```python
from build123d import *

# Parameters (mm, degrees)
F0_R     = 9.5
F1_DEPTH = 10


with BuildPart() as f1:
    # F0 (on Top) → F1 (new body)
    with BuildSketch(Plane.XY):
        with BuildLine():
            Line((0.545393, 36.038877), (-22.02152, 29.448028))
            ThreePointArc((-22.02152, 29.448028), (-26.833244, 26.063712), (-28.572816, 20.444089))
            Line((-28.572816, 20.444089), (-27.988367, 0.026176))
            ThreePointArc((-27.988367, 0.026176), (-27.827538, -1.655225), (-27.444354, -3.300261))
            Line((-27.444354, -3.300261), (-21.763491, -21.955443))
            ThreePointArc((-21.763491, -21.955443), (-21.078383, -23.186097), (-19.947006, -24.025066))
            Line((-19.947006, -24.025066), (-0.808983, -32.702572))
            ThreePointArc((-0.808983, -32.702572), (1.170286, -33.37879), (3.242493, -33.662925))
            Line((3.242493, -33.662925), (22.94121, -34.447196))
            ThreePointArc((22.94121, -34.447196), (23.121499, -34.452579), (23.30186, -34.454373))
            Line((23.30186, -34.454373), (30.367569, -34.454373))
            ThreePointArc((30.367569, -34.454373), (31.781783, -33.868586), (32.367569, -32.454373))
            Line((32.367569, -32.454373), (32.367569, -25.388663))
            ThreePointArc((32.367569, -25.388663), (29.712285, -18.978239), (23.30186, -16.322954))
            Line((23.30186, -16.322954), (21.110382, -16.322954))
            ThreePointArc((21.110382, -16.322954), (19.342615, -15.590721), (18.610382, -13.822954))
            Line((18.610382, -13.822954), (18.610382, 19.213525))
            Line((18.610382, 19.213525), (17.989468, 21.163003))
            ThreePointArc((17.989468, 21.163003), (16.488271, 24.335084), (14.202401, 26.99788))
            Line((14.202401, 26.99788), (5.242804, 34.979598))
            ThreePointArc((5.242804, 34.979598), (3.031016, 36.116406), (0.545393, 36.038877))
        make_face()
        with Locations((-1.962485, -6.192283)):
            Circle(F0_R, mode=Mode.SUBTRACT)
        with BuildLine():
            ThreePointArc((18.80186, -23.888663), (23.30186, -19.388663), (27.80186, -23.888663))
            Line((27.80186, -23.888663), (27.80186, -26.888663))
            ThreePointArc((27.80186, -26.888663), (23.30186, -31.388663), (18.80186, -26.888663))
            Line((18.80186, -26.888663), (18.80186, -23.888663))
        make_face(mode=Mode.SUBTRACT)
        with BuildLine():
            ThreePointArc((-23.967964, 22.20471), (-19.467964, 26.70471), (-14.967964, 22.20471))
            Line((-14.967964, 22.20471), (-14.967964, 19.20471))
            ThreePointArc((-14.967964, 19.20471), (-19.467964, 14.70471), (-23.967964, 19.20471))
            Line((-23.967964, 19.20471), (-23.967964, 22.20471))
        make_face(mode=Mode.SUBTRACT)
    extrude(amount=F1_DEPTH)


solid = f1.part
```
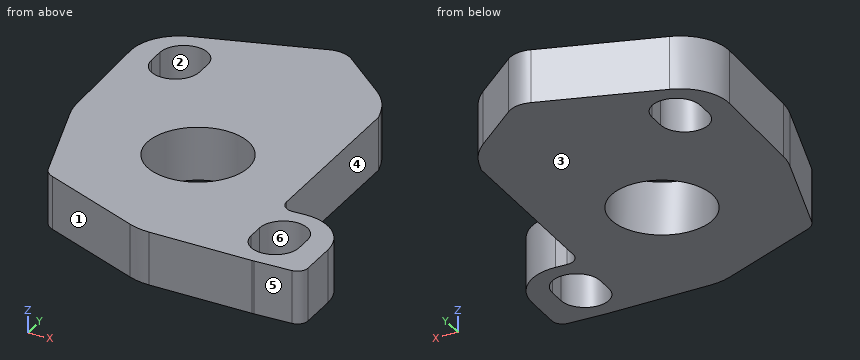
Source: CAD feature listing. Evaluate the final solid. Frame: model axes, mm. Face numbers are marked on the shaded views. A direction names the side the tool comes from. Round coordinates to 2 decimals unless told otherwise and drop trailing zeros. Loops run counter-clockwise (first coordinate to the right, second up) from the corner with the lowest first, then second, coordinate; pieces in that order, holes last. Notation, with made-up numbers: M -20,26 L -10,26 A30 cw -10,56 Z; hole C -3.5,62 d7. An arc over 180 degrees is marked long. Use a Markdown table: item, result. Add a question column.
1. Ray query, line 1 along X through (y, z) = (-4.5, 5); line 2 along X through (y, z) = (25, 8); line 3 along Y through (x, z) = (24, 4.25). Return the intervals inside material, ascending. Write a range as [from, to].
2. Cut plane A-A, the plane x = -8.5. Output: boundary loops of the cut face in (y, z), and give its area (3 significant figures).
3. Pull-direction query (X, two-part tool) for the marked faces 1, 2, 3 and 4; classes: +X half, -X half, draft (parallel to the pull), parting line (faces both ways), or undercut.
4. Cut plane D-D, the plane y = 7. Output: boundary loops of the cut face in (x, z), and give its area (3 significant figures).
5. Cut plane B-B, the plane y = -7.5. Output: boundary loops of the cut face in (x, z).
6. Contact query for flat-ended pins moving along their axis: pin 1 (3 mm diameter, centred on x = -15, z = 8, fed in from -Y); pin 2 (0.9 mm diameter, centred on y = -26, z = 3, fed in from -X); pin 3 (0.9 mm diameter, centred on y = 21.5, z = 6.5, fed in from +X); pin 4 (17 mm diameter, centred on x = -1.96, y = -6.19, fed in from +Z). Output: stop coordinate, or through.
7. Set-up query: the marked faces 5 and 6. Return all of +Z, -Z, +X, -X, +Y, -Y with unobstructed straight access to the full face (end or side cutting, diameter ignored); none if empty.
8. Cut plane C-C, the plane z = 9. State how many separate pieces and enclosed holes the cut face has, and give its area (3 significant figures).
Solution:
| question | item | result |
|---|---|---|
| 1 | line 1 | x = [-27.08, -11.31], [7.39, 18.61] |
| 1 | line 2 | x = [-27.5, -22.99], [-15.94, 16.03] |
| 1 | line 3 | y = [-34.45, -31.33], [-19.44, -16.35] |
| 2 | outline | M -29.22,0 L -13.09,0 L -13.09,10 L -29.22,10 Z; M 0.7,0 L 33.4,0 L 33.4,10 L 0.7,10 Z |
| 2 | area | 488 mm2 |
| 3 | face 1 | -X half |
| 3 | face 2 | undercut |
| 3 | face 3 | draft |
| 3 | face 4 | +X half |
| 4 | outline | M -28.19,0 L 18.61,0 L 18.61,10 L -28.19,10 Z |
| 4 | area | 468 mm2 |
| 5 | outline | M -26.17,0 L -11.37,0 L -11.37,10 L -26.17,10 Z; M 7.45,0 L 18.61,0 L 18.61,10 L 7.45,10 Z |
| 6 | pin 1 | stops at y = -26.95 |
| 6 | pin 2 | stops at x = -16.58 |
| 6 | pin 3 | stops at x = 18.03 |
| 6 | pin 4 | passes through |
| 7 | face 5 | +Z, -Z, +X, -X, -Y |
| 7 | face 6 | +Z, -Z |
| 8 | separate pieces | 1 |
| 8 | enclosed holes | 3 |
| 8 | area | 2,550 mm2 |
